Input: part model. Units: mm. Frame: model coordinates. A direction names the side the tool comes from. Coordinates: 2 decimals unless noted, no trailing zeros. Order: outer loops, then holes, each group sorted by start corner. A loop starts at its lowest first (then second) coordinate and runs counter-clockwise, first axis right, second up.
from build123d import *

# Parameters (mm, degrees)
BOSS_EXTRUDE1_DEPTH    = 8
SKETCH2_W              = 45
SKETCH2_H              = 52
CUT_EXTRUDE1_DEPTH     = 342.206659287
SPLIT1_SURFACE_1_BACK  = 343.199
SPLIT1_SURFACE_1_DEPTH = 686.398
SPLIT1_SURFACE_2_BACK  = 343.199
SPLIT1_SURFACE_2_DEPTH = 686.398
SKETCH5_R              = 2.5
CUT_EXTRUDE6_DEPTH     = 5.2
SKETCH4_R              = 2.5
CUT_EXTRUDE7_DEPTH     = 5.2
SKETCH6_R              = 2.5
CUT_EXTRUDE8_DEPTH     = 184.408541223


with BuildPart() as part:
    # Sketch1 → Boss-Extrude1 (new body)
    with BuildSketch(Plane.XY):
        with BuildLine():
            Line((70, 309.985818768), (85.299227191, 309.985818768))
            ThreePointArc((85.299227191, 309.985818768), (88.489017574, 308.836174247), (90.211957942, 305.915913694))
            Line((90.211957942, 305.915913694), (96.672728921, 271.790334282))
            ThreePointArc((96.672728921, 271.790334282), (97.06575438, 270.906904614), (97.621470019, 270.115641625))
            Line((97.621470019, 270.115641625), (139.950460317, 220.786053348))
            ThreePointArc((139.950460317, 220.786053348), (141.739336996, 217.746026552), (142.361429131, 214.274017901))
            Line((142.361429131, 214.274017901), (142.361429131, 30.859943174))
            ThreePointArc((142.361429131, 30.859943174), (140.896963037, 27.324409268), (137.361429131, 25.859943174))
            Line((137.361429131, 25.859943174), (114.717190871, 25.782318449))
            ThreePointArc((114.717190871, 25.782318449), (112.681998989, 25.341726514), (111.002773989, 24.110332733))
            Line((111.002773989, 24.110332733), (89.38285929, 0))
            Line((89.38285929, 0), (50.5, 0))
            Line((50.5, 0), (28.997226011, 24.110332733))
            ThreePointArc((28.997226011, 24.110332733), (27.318001011, 25.341726514), (25.282809129, 25.782318449))
            Line((25.282809129, 25.782318449), (2.638570869, 25.859943174))
            ThreePointArc((2.638570869, 25.859943174), (-0.896963037, 27.324409268), (-2.361429131, 30.859943174))
            Line((-2.361429131, 30.859943174), (-2.361429131, 214.274017901))
            ThreePointArc((-2.361429131, 214.274017901), (-1.739336996, 217.746026552), (0.049539683, 220.786053348))
            Line((0.049539683, 220.786053348), (42.261389271, 270.115641625))
            ThreePointArc((42.261389271, 270.115641625), (42.81710491, 270.906904614), (43.210130369, 271.790334282))
            Line((43.210130369, 271.790334282), (49.724618218, 305.923183314))
            ThreePointArc((49.724618218, 305.923183314), (51.449026762, 308.838533573), (54.635967087, 309.985818768))
            Line((54.635967087, 309.985818768), (70, 309.985818768))
        make_face()
        with BuildLine():
            Line((12.638570869, 35.492492662), (15.638570869, 35.492492662))
            ThreePointArc((15.638570869, 35.492492662), (19.174104775, 36.956958756), (20.638570869, 40.492492662))
            Line((20.638570869, 40.492492662), (20.638570869, 213.625959477))
            Line((20.638570869, 213.625959477), (7.638570869, 213.625959477))
            Line((7.638570869, 213.625959477), (7.638570869, 40.492492662))
            ThreePointArc((7.638570869, 40.492492662), (9.103036963, 36.956958756), (12.638570869, 35.492492662))
        make_face(mode=Mode.SUBTRACT)
        with BuildLine():
            Line((127.361429131, 35.492492662), (124.361429131, 35.492492662))
            ThreePointArc((124.361429131, 35.492492662), (120.825895225, 36.956958756), (119.361429131, 40.492492662))
            Line((119.361429131, 40.492492662), (119.361429131, 213.625959477))
            Line((119.361429131, 213.625959477), (132.361429131, 213.625959477))
            Line((132.361429131, 213.625959477), (132.361429131, 40.492492662))
            ThreePointArc((132.361429131, 40.492492662), (130.896963037, 36.956958756), (127.361429131, 35.492492662))
        make_face(mode=Mode.SUBTRACT)
    extrude(amount=BOSS_EXTRUDE1_DEPTH)

    # Sketch2 → Cut-Extrude1 (cut, through all)
    with BuildSketch(Plane.XY.offset(8)):
        with Locations((69.88285929, 180.008918923)):
            Rectangle(SKETCH2_W, SKETCH2_H)
    extrude(amount=-CUT_EXTRUDE1_DEPTH, mode=Mode.SUBTRACT)


with BuildPart() as body_2:
    # Split1: the piece behind the surface
    add(part.part)
    # Split1 surface: a surface, the sketch's curves swept straight by 686.398 mm
    with BuildLine(Plane(origin=(0, 0, 0), x_dir=(-1, 0, 0), z_dir=(0, 0, -1)).offset(-SPLIT1_SURFACE_1_BACK), mode=Mode.PRIVATE) as split1_surface_1_path:
        Line((-142.361429131, 115.359943174), (2.361429131, 115.359943174))
    split1_surface_1 = Shell.extrude(split1_surface_1_path.wire(), (0 * SPLIT1_SURFACE_1_DEPTH, 0 * SPLIT1_SURFACE_1_DEPTH, -1 * SPLIT1_SURFACE_1_DEPTH))
    split(bisect_by=split1_surface_1, keep=Keep.BOTTOM)

    # Sketch5 → Cut-Extrude6 (cut)
    with BuildSketch(Plane(origin=(0, 115.359943174, -115.359943174), x_dir=(1, 0, 0), z_dir=(0, -1, 0))):
        with Locations(Location((100, 119.359943174, 0), (0, 0, 90))):
            Circle(SKETCH5_R)
        with Locations(Location((2.638570869, 119.359943174, 0), (0, 0, 270))):
            Circle(SKETCH5_R)
        with Locations(Location((40, 119.359943174, 0), (0, 0, 270))):
            Circle(SKETCH5_R)
        with Locations(Location((70, 119.359943174, 0), (0, 0, 270))):
            Circle(SKETCH5_R)
        with Locations(Location((137.361429131, 119.359943174, 0), (0, 0, 270))):
            Circle(SKETCH5_R)
    extrude(amount=CUT_EXTRUDE6_DEPTH, mode=Mode.SUBTRACT)

    # Sketch6 → Cut-Extrude8 (cut, through all)
    with BuildSketch(Plane.XY.offset(8)):
        with Locations((37.078570869, 81.192492662)):
            Circle(SKETCH6_R)
        with Locations((104.078570869, 81.192492662)):
            Circle(SKETCH6_R)
        with Locations((104.078570869, 41.192492662)):
            Circle(SKETCH6_R)
        with Locations((37.078570869, 41.192492662)):
            Circle(SKETCH6_R)
    extrude(amount=-CUT_EXTRUDE8_DEPTH, mode=Mode.SUBTRACT)


with BuildPart() as part_1:
    add(part.part)

    # Split1: split by a surface, the side it looks to stays
    # Split1 surface: a surface, the sketch's curves swept straight by 686.398 mm
    with BuildLine(Plane(origin=(0, 0, 0), x_dir=(-1, 0, 0), z_dir=(0, 0, -1)).offset(-SPLIT1_SURFACE_2_BACK), mode=Mode.PRIVATE) as split1_surface_2_path:
        Line((-142.361429131, 115.359943174), (2.361429131, 115.359943174))
    split1_surface_2 = Shell.extrude(split1_surface_2_path.wire(), (0 * SPLIT1_SURFACE_2_DEPTH, 0 * SPLIT1_SURFACE_2_DEPTH, -1 * SPLIT1_SURFACE_2_DEPTH))
    split(bisect_by=split1_surface_2, keep=Keep.TOP)

    # Sketch4 → Cut-Extrude7 (cut)
    with BuildSketch(Plane(origin=(0, 115.359943174, 0), x_dir=(-1, 0, 0), z_dir=(0, -1, 0))):
        with Locations(Location((-70, -4, 0), (0, 0, 90))):
            Circle(SKETCH4_R)
        with Locations(Location((-40, -4, 0), (0, 0, 90))):
            Circle(SKETCH4_R)
        with Locations(Location((-100, -4, 0), (0, 0, 270))):
            Circle(SKETCH4_R)
        with Locations(Location((-137.361429131, -4, 0), (0, 0, 90))):
            Circle(SKETCH4_R)
        with Locations(Location((-2.638570869, -4, 0), (0, 0, 90))):
            Circle(SKETCH4_R)
    extrude(amount=-CUT_EXTRUDE7_DEPTH, mode=Mode.SUBTRACT)


solid = body_2.part
Item 1: Cut plane A-A on y = 58.5. Return loops of the section in (x, z), then the cut area to 3 significant figures.
Response values:
outline: (-2.36, 0) - (7.64, 0) - (7.64, 8) - (-2.36, 8) - close; (20.64, 0) - (119.36, 0) - (119.36, 8) - (20.64, 8) - close; (132.36, 0) - (142.36, 0) - (142.36, 8) - (132.36, 8) - close
area: 950 mm2
Item 2: Access query for faces 1 (the face through (119.361, 77, 4)), 2 (the face through (-0.86, 27.29, 3.94)), 3 (the face through (97.52, 112.8, 3.67)). Directions: +Z, -Z, +X, -X, +Y, -Y. A direction counts if a zero-diameter tool reaches every point of the face in a straight line with its end or side. Return the directions, or none.
Response values:
face 1: +Z, -Z, +Y
face 2: +Z, -Z, -X, -Y
face 3: +Y
Item 3: Cut plane B-B on x = 70. Return loops of the section in (y, z).
Response values:
outline: (0, 0) - (115.36, 0) - (115.36, 1.5) - (110.16, 1.5) - (110.16, 6.5) - (115.36, 6.5) - (115.36, 8) - (0, 8) - close
Item 4: Cut plane D-D on z = 4. Count the separate pieces of the cut face and the enclosed holes in it, then the cut area to 3 significant figures.
Response values:
separate pieces: 1
enclosed holes: 4
area: 12,300 mm2
Item 5: Cut plane C-C on y = 37. Return loops of the section in (x, z).
Response values:
outline: (-2.36, 0) - (9.06, 0) - (9.06, 8) - (-2.36, 8) - close; (19.22, 0) - (120.78, 0) - (120.78, 8) - (19.22, 8) - close; (130.94, 0) - (142.36, 0) - (142.36, 8) - (130.94, 8) - close
Item 6: Ray query, probe 1 along X at (y, z) = (69, 1.5); probe 2 along Y at (x, z) = (38, 3); probe 3 along Y at (x, z) = (5, 5.5). Return the intervals inside material, ascending.
Response values:
probe 1: x = -2.36 to 7.64, 20.64 to 119.36, 132.36 to 142.36
probe 2: y = 14.02 to 38.87, 43.52 to 78.87, 83.52 to 110.16
probe 3: y = 25.85 to 115.36
Item 7: Pin query (flat end, axial travel): pin 1 Ø3 at (x, z) = (70, 4) entering from -Y; pin 2 Ø1.5 at (x, z) = (41, 3.5) entering from +Y; pin 3 Ø3 at (x, z) = (2.64, 4) entering from -Y; pin 4 Ø4 at (x, z) = (112, 5.5) entering from -Y. Return the tip coordinate at first contact, or that it passes through.
Response values:
pin 1: stops at y = 0
pin 2: stops at y = 110.16
pin 3: stops at y = 25.85
pin 4: stops at y = 22.99
